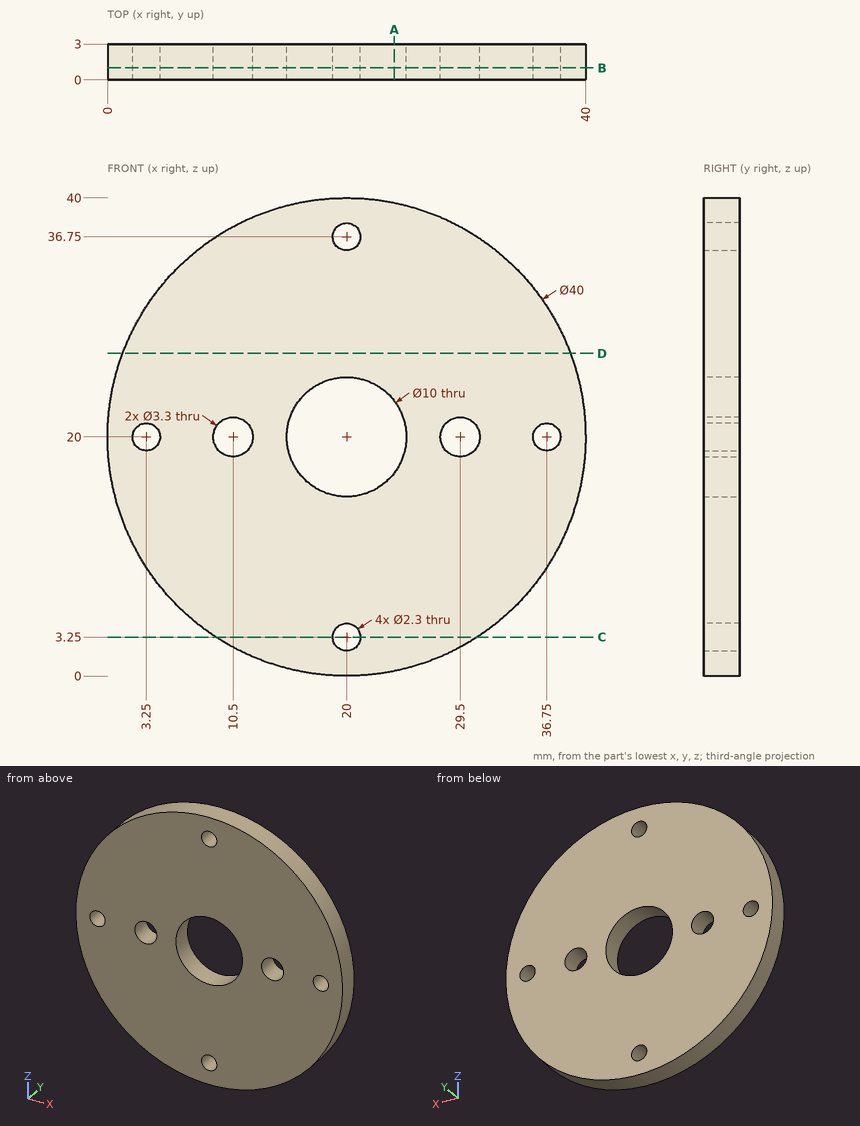
Input: dimensioned drawing with shaded views. Units: mm. Origin: part minimum x, y, z. Round coordinates to 2 decimals unless told otherwise and drop trailing zeros. Loops run counter-clockwise (first coordinate to the right, second up) from the corner with the lowest first, then second, coordinate; pieces in that order, holes last. Notation, with made-up numbers: M 36.5,-24.5 L 53.5,-24.5 A17 cw 53.5,-13.5 Z; hole C -10.75,49 d6. An arc over 180 degrees is marked long. Return JSON: item names as keys, results as strings. Group by question number.
1. Material intervals for line 1 along X through (y, z) = (1, 20); line 2 along X through (y, z) = (0.9, 21); line 3 along X through (y, z) = (1.9, 37), sorted ascending. Write a range as from..to.
2. Section query B-B on y = 1. Output: boundary loops of the cut face in (x, z), and give its area (3 significant figures).
3. Section query D-D on z = 27. Output: boundary loops of the cut face in (x, y) (3 decimals), and give its area (3 significant figures).
4. Section query A-A on x = 24. Output: boundary loops of the cut face in (y, z), and give its area (3 significant figures).
5. Pin query (flat end, axial travel): pin 1 (1.4 mm diameter, centred on x = 3.25, z = 20, fed in from -Y); pin 2 (1.5 mm diameter, centred on y = 0.5, z = 13.5, fed in from -X). Return the tip coordinate at first contact, or that it passes through.
6. Section query C-C on z = 3.25. Output: boundary loops of the cut face in (x, y), and give its area (3 significant figures).
Checks:
{
 "1": {"line 1": "x = 0..2.1, 4.4..8.85, 12.15..15, 25..27.85, 31.15..35.6, 37.9..40", "line 2": "x = 0.03..2.68, 3.82..9.19, 11.81..15.1, 24.9..28.19, 30.81..36.18, 37.32..39.97", "line 3": "x = 9.46..18.88, 21.12..30.54"},
 "2": {"outline": "C 20,20 d40; hole C 3.25,20 d2.3; hole C 10.5,20 d3.3; hole C 20,20 d10; hole C 20,3.25 d2.3; hole C 20,36.75 d2.3; hole C 29.5,20 d3.3; hole C 36.75,20 d2.3", "area": "1,140 mm²"},
 "3": {"outline": "M 1.265,0 L 38.735,0 L 38.735,3 L 1.265,3 Z", "area": "112 mm²"},
 "4": {"outline": "M 0,0.4 L 3,0.4 L 3,17 L 0,17 Z; M 0,23 L 3,23 L 3,39.6 L 0,39.6 Z", "area": "99.6 mm²"},
 "5": {"pin 1": "passes through", "pin 2": "stops at x = 0.84"},
 "6": {"outline": "M 9.07,0 L 18.85,0 L 18.85,3 L 9.07,3 Z; M 21.15,0 L 30.93,0 L 30.93,3 L 21.15,3 Z", "area": "58.7 mm²"}
}
